from build123d import *

# Parameters (mm, degrees)
PAD005_DEPTH     = 4
PAD002_DEPTH     = 1
PAD003_DEPTH     = 3
HOLE_D           = 3.5
HOLE_CBORE_D     = 6
HOLE_CBORE_DEPTH = 2
SKETCH011_R      = 2.5
SKETCH011_W      = 9.042401
SKETCH011_H      = 3.767665
SKETCH011_W_2    = 24
SKETCH011_H_2    = 3
SKETCH011_W_3    = 1.5
SKETCH011_H_3    = 2.5
POCKET005_DEPTH  = 5
SKETCH012_W      = 5.629994
SKETCH012_H      = 16.889996
SKETCH012_W_2    = 13.176597
SKETCH012_H_2    = 7.067448
POCKET006_DEPTH  = 0.5


with BuildPart() as usb_c_cutter:
    # Sketch008 → Pad005 (new body)
    with BuildSketch(Plane(origin=(0, 0, 0), x_dir=(0, -1, 0), z_dir=(-1, 0, 0))):
        with BuildLine():
            Line((2.535801, 11.911979), (12.347588, 11.911979))
            ThreePointArc((14.347588, 9.911979), (13.761802, 11.326192), (12.347588, 11.911979))
            Line((14.347588, 9.911979), (14.347588, 3.866895))
            ThreePointArc((12.347588, 1.866895), (13.761802, 2.452682), (14.347588, 3.866895))
            Line((12.347588, 1.866895), (2.535801, 1.866895))
            ThreePointArc((0.535801, 3.866895), (1.121588, 2.452682), (2.535801, 1.866895))
            Line((0.535801, 3.866895), (0.535801, 9.911979))
            ThreePointArc((2.535801, 11.911979), (1.121588, 11.326192), (0.535801, 9.911979))
        make_face()
    extrude(amount=-PAD005_DEPTH)


with BuildPart() as usb_c_cutter_1:
    # Body002 placement: moved
    add(usb_c_cutter.part.moved(Location((-26, 0, 0))))


with BuildPart() as lid_pocketed:
    # Sketch005 → Pad002 (new body)
    with BuildSketch(Plane.XY.offset(7)):
        with BuildLine():
            Line((-20.15, 23.75), (20.15, 23.75))
            ThreePointArc((23.75, 20.15), (22.695584, 22.695584), (20.15, 23.75))
            Line((23.75, 20.15), (23.75, -20.15))
            ThreePointArc((20.15, -23.75), (22.695584, -22.695584), (23.75, -20.15))
            Line((20.15, -23.75), (-20.15, -23.75))
            ThreePointArc((-23.75, -20.15), (-22.695584, -22.695584), (-20.15, -23.75))
            Line((-23.75, -20.15), (-23.75, 20.15))
            ThreePointArc((-20.15, 23.75), (-22.695584, 22.695584), (-23.75, 20.15))
        make_face()
    extrude(amount=PAD002_DEPTH)

    # Sketch006 (on Face10 of Pad002) → Pad003 (join)
    with BuildSketch(Plane.XY.offset(8)):
        with BuildLine():
            Line((-20.2, 25.5), (20.2, 25.5))
            ThreePointArc((25.5, 20.2), (23.947666, 23.947666), (20.2, 25.5))
            Line((25.5, 20.2), (25.5, -20.2))
            ThreePointArc((20.2, -25.5), (23.947666, -23.947666), (25.5, -20.2))
            Line((20.2, -25.5), (-20.2, -25.5))
            ThreePointArc((-25.5, -20.2), (-23.947666, -23.947666), (-20.2, -25.5))
            Line((-25.5, -20.2), (-25.5, 20.2))
            ThreePointArc((-20.2, 25.5), (-23.947666, 23.947666), (-25.5, 20.2))
        make_face()
    extrude(amount=PAD003_DEPTH)

    # Hole (through all)
    with Locations(Plane.XY.offset(11)):
        with Locations((-20, 20), (20, 20), (20, -20), (-20, -20)):
            CounterBoreHole(HOLE_D / 2, HOLE_CBORE_D / 2, HOLE_CBORE_DEPTH)


with BuildPart() as lid_pocketed_1:
    # Body001 placement: moved
    add(lid_pocketed.part.moved(Location((0, 0, 2))))

    # Cut: cut USB-C Cutter
    add(usb_c_cutter_1.part, mode=Mode.SUBTRACT)

    # Sketch011 (on Face7 of BaseFeature001) → Pocket005 (cut)
    with BuildSketch(Plane.XY.offset(13)):
        with Locations((-14.102295, 19.26004)):
            Circle(SKETCH011_R)
        with Locations((8.547714, 14.450916)):
            Rectangle(SKETCH011_W, SKETCH011_H)
        Polygon((15.998645, 16.994311), (21.498645, 16.994311), (21.498645, 5.994311), (20.28048, 5.994311), (20.28048, -15.505689), (17.5, -15.505689), (17.5, -22.047392), (2.5, -22.047392), (2.5, -20.535681), (-9.5, -20.535681), (-9.5, -14.535681), (2.5, -14.535681), (2.5, -13.047392), (17.5, -13.047392), (17.5, 5.994311), (15.998645, 5.994311), align=None)
        with Locations((3.585587, 19.303802)):
            Rectangle(SKETCH011_W_2, SKETCH011_H_2)
        with Locations((-1.504905, 14.45)):
            Rectangle(SKETCH011_W_3, SKETCH011_H_3)
        with Locations((1.020606, 14.45)):
            Rectangle(SKETCH011_W_3, SKETCH011_H_3)
        with Locations((0.989071, 8.45)):
            Rectangle(SKETCH011_W_3, SKETCH011_H_3)
        with Locations((-1.499158, 8.45)):
            Rectangle(SKETCH011_W_3, SKETCH011_H_3)
        with Locations((-4.069136, 8.45)):
            Rectangle(SKETCH011_W_3, SKETCH011_H_3)
    extrude(amount=-POCKET005_DEPTH, mode=Mode.SUBTRACT)

    # Sketch012 (on Face76 of Pocket005) → Pocket006 (cut)
    with BuildSketch(Plane(origin=(0, 0, 9), x_dir=(1, 0, 0), z_dir=(0, 0, -1))):
        with Locations((-18.033425, -7.323527)):
            Rectangle(SKETCH012_W, SKETCH012_H)
        with Locations((8.540513, -14.609106)):
            Rectangle(SKETCH012_W_2, SKETCH012_H_2)
    extrude(amount=-POCKET006_DEPTH, mode=Mode.SUBTRACT)


solid = lid_pocketed_1.part
Read the model definition and answer for the solid it produces. Units are mm, in the model's axes. A direction names the side the tool comes from. Round coordinates to 2 decimals unless told otherwise and drop trailing zeros. Write each loop counter-clockwise with the first axis right and the second up, starting at its lowest first coordinate (ties: lowest second). Pieces come first, ordered by that corner, then holes.
1. Determine the mould class of faces 1 (the face through (-23.906, 23.989, 11.479)), 2 (the face through (-20, 18, 11)), 3 (the face through (23.906, -23.989, 11.479)), 4 (the face through (1, 15.7, 11)) for opening direction Y: pulls with the +Y half, pulls with the -Y half, needs draft (parallel to the pull), parting line crosses it, or undercut.
2. The part is cut by section C-C, the plane y = -11. Determine the outline of the cut face in (x, z), then the cut area to 3 significant figures.
3. The part is cut by section B-B, the plane x = 10. Determine the outline of the cut face in (y, z).
4. The part is cut by section A-A, the plane y = 15. State how many separate pieces and enclosed holes the cut face has, then the cut area to 3 significant figures.
5. Straight lines are drawn through the part: L1, parallel to Y at x = 13, z = 11.4; L2, parallel to Y at x = -20, z = 10.5; L3, parallel to Y at x = 20, z = 10.15. For each, find the intervals that lie inside material, in ascending order.
6. Which of the six approach directions +Z, -Z, +X, -X, +Y, -Y give full straight-line access (tool end or side, diameter ignored) to faces 5 (the face through (-0.755, 14, 11)), 6 (the face through (22.72, 22.67, 9.49)), 7 (the face through (-22, -8, 10))?
7. Given pin 1 Ø4.5 at (x, y) = (-18.5, 4) entering from -Z; pin 2 Ø0.8 at (y, z) = (-1.5, 9.5) entering from +X, each flat-ended and moving along its own axis, determine where each tip first touches the part or whether it passes through.
8. The part is cut by section D-D, the plane y = -19. Determine the outline of the cut face in (x, z), then the cut area to 3 significant figures.
Values:
1. face 1: pulls with the +Y half
1. face 2: undercut
1. face 3: pulls with the -Y half
1. face 4: undercut
2. outline: (-25.5, 11.91) - (-22, 11.91) - (-22, 9) - (17.5, 9) - (17.5, 13) - (-25.5, 13) - close; (20.28, 9) - (23.75, 9) - (23.75, 10) - (25.5, 10) - (25.5, 13) - (20.28, 13) - close
2. area: 181 mm2
3. outline: (-25.5, 10) - (-23.75, 10) - (-23.75, 9) - (-22.05, 9) - (-22.05, 13) - (-25.5, 13) - close; (-13.05, 9) - (11.08, 9) - (11.08, 9.5) - (12.57, 9.5) - (12.57, 13) - (-13.05, 13) - close; (16.33, 9.5) - (17.8, 9.5) - (17.8, 13) - (16.33, 13) - close; (20.8, 9) - (23.75, 9) - (23.75, 10) - (25.5, 10) - (25.5, 13) - (20.8, 13) - close
4. separate pieces: 5
4. enclosed holes: 0
4. area: 125 mm2
5. L1: y = -25.5 to -22.05, -13.05 to 12.57, 16.33 to 17.8, 20.8 to 25.5
5. L2: y = -25.5 to -21.75, -18.25 to 18.25, 21.75 to 25.5
5. L3: y = -25.5 to -21.75, -18.25 to -15.51, 16.99 to 18.25, 21.75 to 25.5
6. face 5: +Z, -Z
6. face 6: -Z, +X, +Y
6. face 7: -Z, -X
7. pin 1: stops at z = 9.5
7. pin 2: stops at x = 23.75
8. outline: (-25.5, 10) - (-23.75, 10) - (-23.75, 9) - (-21.44, 9) - (-21.44, 11) - (-22.83, 11) - (-22.83, 13) - (-25.5, 13) - close; (-18.56, 9) - (-9.5, 9) - (-9.5, 13) - (-17.17, 13) - (-17.17, 11) - (-18.56, 11) - close; (17.5, 9) - (18.56, 9) - (18.56, 11) - (17.5, 11) - close; (21.44, 9) - (23.75, 9) - (23.75, 10) - (25.5, 10) - (25.5, 13) - (22.83, 13) - (22.83, 11) - (21.44, 11) - close
8. area: 59.0 mm2
